Geometry check sheet. Reference: the model listing, model coordinates, mm. Face numbers are marked on the shaded views. A direction names the side the tool comes from. Round coordinates to 2 decimals unless told otherwise and drop trailing zeros. Order: outer loops, then holes, each group sorted by start corner. A loop starts at its lowest first (then second) coordinate and runs counter-clockwise, first axis right, second up. Notation, with made-up numbers: (74, 74.5) - (94, 74.5) arc R23 cw to (94, 102.5) - close; hole circle Ø4 at (4, 40.5). An arc over 180 degrees is marked (long way). One line per question, with ' | ' between items. Start each with the question number.
Q1. Tool access check on the marked faces 1, 2 and 3. Record the directions out of +Z, -Z, +X, -X, +Y, -Y that give a thin tool (end or side, any length) a straight path to the whole face; none if there is none.
Q2. Gauge pin test, flat ends, axial feed: P1, Ø9.5, axis at x = 0, y = 0, coming from the -Z side; P2, Ø0.9, axis at y = 7.5, z = 1.5, coming from the -X side; P3, Ø3, axis at x = -5.17, y = 8.85, coming from the +Z side; P4, Ø5, axis at x = 0, y = 0, coming from the +Z side. Record the tip position at first contact, or that the pin passes through.
Q3. Material ranges on line 1 along Y through (x, z) = (0, 2.8); line 2 along Y through (x, z) = (0, 0.3); line 3 along X through (y, z) = (-10.5, 2.75), recorded low to high.
Q4. Sectioned sample at B-B, the plane y = -17.5. Enter the section's corners in (x, z), then the cut area to 3 significant figures.
Q5. Sectioned sample at D-D, the plane y = 0. Give the number of separate pieces and of enclosed holes in the cut face, then the cut area to 3 significant figures.
Q6. Sectioned sample at A-A, the plane x = 0. Enter the section's corners in (y, z).
Q7. Sectioned sample at C-C, the plane z = 1.85. Enter the section's corners in (x, y) (3 decimals).
Q8. Mould release check, pull along Y, two halves, no side actions. Record for the marked faces 4, 5, 6 and 7: +Y half, -Y half, draft (parallel to the pull), parting line (faces both ways), or undercut.
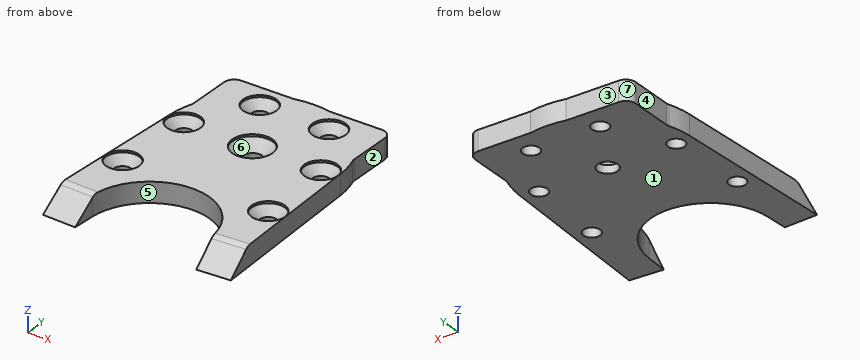
```python
from build123d import *

# Parameters (mm, degrees)
SKETCH1_R                                      = 1.25
SKETCH1_R_2                                    = 1.5
BOSS_EXTRUDE1_DEPTH                            = 3
CSK_FOR_M2_5_FLAT_HEAD_MACHINE_SCREW2_AT_COUNT = 2
CSK_FOR_M2_5_FLAT_HEAD_MACHINE_SCREW2_AT_PITCH = 10.201972061
CSK_FOR_M2_5_FLAT_HEAD_MACHINE_SCREW_2_COUNT   = 2
CSK_FOR_M2_5_FLAT_HEAD_MACHINE_SCREW_2_PITCH   = 17.781163237
CSK_FOR_M2_5_FLAT_HEAD_MACHINE_SCREW_3_COUNT   = 2
CSK_FOR_M2_5_FLAT_HEAD_MACHINE_SCREW_3_PITCH   = 20.5
CSK_FOR_M2_5_FLAT_HEAD_MACHINE_SCREW_4_COUNT   = 2
CSK_FOR_M2_5_FLAT_HEAD_MACHINE_SCREW_4_PITCH   = 12
CSK_FOR_M2_5_FLAT_HEAD_MACHINE_SCREW_5_COUNT   = 2
CSK_FOR_M2_5_FLAT_HEAD_MACHINE_SCREW_5_PITCH   = 24.295707673
CUT_EXTRUDE4_REACH                             = 38.909
CUT_EXTRUDE5_REACH                             = 38.909
FILLET2_R                                      = 1.5


with BuildPart() as part:
    # Sketch1 → Boss-Extrude1 (new body)
    with BuildSketch(Plane.XY):
        with BuildLine():
            ThreePointArc((12.078947368, 4.081853803), (12.019868427, 4.318739766), (12, 4.562071898))
            Line((12, 4.562071898), (12, 10.970231229))
            ThreePointArc((12, 10.970231229), (11.560660172, 12.030891401), (10.5, 12.470231229))
            Line((10.5, 12.470231229), (2.656281818, 12.470231229))
            ThreePointArc((2.656281818, 12.470231229), (0, 12.75), (-2.656281818, 12.470231229))
            Line((-2.656281818, 12.470231229), (-10.5, 12.470231229))
            ThreePointArc((-10.5, 12.470231229), (-11.560660172, 12.030891401), (-12, 10.970231229))
            Line((-12, 10.970231229), (-12, 4.562071898))
            ThreePointArc((-12, 4.562071898), (-12.019868427, 4.318739766), (-12.078947368, 4.081853803))
            ThreePointArc((-12.078947368, 4.081853803), (-12.522664749, 2.396949642), (-12.732526568, 0.667283442))
            Line((-12.732526568, 0.667283442), (-14.040925474, -24.298454927))
            Line((-14.040925474, -24.298454927), (-9.0477778, -24.560134708))
            Line((-9.0477778, -24.560134708), (-8.869966, -21.167283442))
            ThreePointArc((-8.869966, -21.167283442), (0, -12.75), (8.869966, -21.167283442))
            Line((8.869966, -21.167283442), (9.0477778, -24.560134708))
            Line((9.0477778, -24.560134708), (14.040925474, -24.298454927))
            Line((14.040925474, -24.298454927), (12.732526568, 0.667283442))
            ThreePointArc((12.732526568, 0.667283442), (12.522664749, 2.396949642), (12.078947368, 4.081853803))
        make_face()
        with Locations((5.172915418, 8.848923442)):
            Circle(SKETCH1_R, mode=Mode.SUBTRACT)
        with Locations((10.25, 0)):
            Circle(SKETCH1_R, mode=Mode.SUBTRACT)
        with Locations((10.884912472, -11.983191818)):
            Circle(SKETCH1_R, mode=Mode.SUBTRACT)
        Circle(SKETCH1_R_2, mode=Mode.SUBTRACT)
        with Locations((-10.25, 0)):
            Circle(SKETCH1_R, mode=Mode.SUBTRACT)
        with Locations((-5.172915418, 8.848923442)):
            Circle(SKETCH1_R, mode=Mode.SUBTRACT)
        with Locations((-10.884912472, -11.983191818)):
            Circle(SKETCH1_R, mode=Mode.SUBTRACT)
    extrude(amount=BOSS_EXTRUDE1_DEPTH)

    # Sketch3 → CSK for M3 Flat Head Machine Screw1 (revolve, cut)
    with BuildSketch(Plane(origin=(0, 0, 3), x_dir=(0, -1, 0), z_dir=(1, 0, 0))):
        Polygon((0, 0), (0, 5.901290929), (1.5, 5), (1.5, 1.8), (3, 0.3), (3, 0), align=None)
    revolve(axis=Axis((0, 0, 9.35), (0, 0, -1)), mode=Mode.SUBTRACT)

    # Sketch6 → CSK for M2.5 Flat Head Machine Screw2 (revolve, cut)
    with BuildSketch(Plane(origin=(-10.25, 0, 3), x_dir=(0, -1, 0), z_dir=(1, 0, 0))):
        Polygon((0, 0), (0, 5.751075774), (1.25, 5), (1.25, 1.525), (2.475, 0.3), (2.475, 0), align=None)
    csk_for_m2_5_flat_head_machine_screw2 = revolve(axis=Axis((-10.25, 0, 9.35), (0, 0, -1)), mode=Mode.SUBTRACT)

    # CSK for M2.5 Flat Head Machine Screw2 at: CSK for M2.5 Flat Head Machine Screw2 ×2
    with Locations(*[Vector(0.4976571736965763, 0.8673738164530538, 0) * (i * CSK_FOR_M2_5_FLAT_HEAD_MACHINE_SCREW2_AT_PITCH) for i in range(1, CSK_FOR_M2_5_FLAT_HEAD_MACHINE_SCREW2_AT_COUNT)]):
        add(csk_for_m2_5_flat_head_machine_screw2, mode=Mode.SUBTRACT)

    # CSK for M2.5 Flat Head Machine Screw 2: CSK for M2.5 Flat Head Machine Screw2 ×2
    with Locations(*[Vector(0.8673738164530539, 0.497657173696576, 0) * (i * CSK_FOR_M2_5_FLAT_HEAD_MACHINE_SCREW_2_PITCH) for i in range(1, CSK_FOR_M2_5_FLAT_HEAD_MACHINE_SCREW_2_COUNT)]):
        add(csk_for_m2_5_flat_head_machine_screw2, mode=Mode.SUBTRACT)

    # CSK for M2.5 Flat Head Machine Screw 3: CSK for M2.5 Flat Head Machine Screw2 ×2
    with Locations(*[(i * CSK_FOR_M2_5_FLAT_HEAD_MACHINE_SCREW_3_PITCH, 0, 0) for i in range(1, CSK_FOR_M2_5_FLAT_HEAD_MACHINE_SCREW_3_COUNT)]):
        add(csk_for_m2_5_flat_head_machine_screw2, mode=Mode.SUBTRACT)

    # CSK for M2.5 Flat Head Machine Screw 4: CSK for M2.5 Flat Head Machine Screw2 ×2
    with Locations(*[Vector(-0.05290937262723391, -0.9985993181893289, 0) * (i * CSK_FOR_M2_5_FLAT_HEAD_MACHINE_SCREW_4_PITCH) for i in range(1, CSK_FOR_M2_5_FLAT_HEAD_MACHINE_SCREW_4_COUNT)]):
        add(csk_for_m2_5_flat_head_machine_screw2, mode=Mode.SUBTRACT)

    # CSK for M2.5 Flat Head Machine Screw 5: CSK for M2.5 Flat Head Machine Screw2 ×2
    with Locations(*[Vector(0.8699031432206916, -0.4932225881027359, 0) * (i * CSK_FOR_M2_5_FLAT_HEAD_MACHINE_SCREW_5_PITCH) for i in range(1, CSK_FOR_M2_5_FLAT_HEAD_MACHINE_SCREW_5_COUNT)]):
        add(csk_for_m2_5_flat_head_machine_screw2, mode=Mode.SUBTRACT)

    # Sketch10 → Cut-Extrude4 (cut, up to next)
    with BuildSketch(Plane(origin=(12.732526568, 0.667283442, 0), x_dir=(0, 0, -1), z_dir=(0.9986295347545739, 0.052335956242944286, 0)), mode=Mode.PRIVATE) as cut_extrude4_sk1:
        Polygon((-3, -25), (0, -25), (-3, -21.113156261), align=None)
    cut_extrude4_tool1 = extrude(cut_extrude4_sk1.sketch, amount=-CUT_EXTRUDE4_REACH, mode=Mode.PRIVATE) & part.part
    add(cut_extrude4_tool1.solids().sort_by_distance((13.973118, -23.004616, 2))[0], mode=Mode.SUBTRACT)

    # Sketch11 → Cut-Extrude5 (cut, up to next)
    with BuildSketch(Plane(origin=(-12.732526568, 0.667283442, 0), x_dir=(0, 0, 1), z_dir=(-0.9986295347545739, 0.052335956242944716, 0)), mode=Mode.PRIVATE) as cut_extrude5_sk1:
        Polygon((3, -21.113156261), (0, -25), (3, -25), align=None)
    cut_extrude5_tool1 = extrude(cut_extrude5_sk1.sketch, amount=-CUT_EXTRUDE5_REACH, mode=Mode.PRIVATE) & part.part
    add(cut_extrude5_tool1.solids().sort_by_distance((-13.973118, -23.004616, 2))[0], mode=Mode.SUBTRACT)

    # Fillet2
    fillet2_edges = [part.edges().sort_by_distance(p)[0] for p in [
        (11.334194425, -20.548130857, 3),
        (-11.334194425, -20.548130857, 3),
    ]]
    fillet(fillet2_edges, radius=FILLET2_R)


solid = part.part
```
Determined:
1) face 1: -Z, +X, -X, +Y, -Y | face 2: +Z, -Z, +X, +Y | face 3: +Z, -Z, -X, +Y
2) P1: stops at z = 0 | P2: stops at x = -12 | P3: stops at z = 1.73 | P4: stops at z = 2.2
3) line 1: y = -12.75 to -3, 3 to 12.75 | line 2: y = -12.75 to -1.5, 1.5 to 12.75 | line 3: x = -13.32 to -12.87, -8.9 to 8.9, 12.87 to 13.32
4) outline: (-13.68, 0) - (-7.86, 0) - (-7.86, 3) - (-13.68, 3) - close; (7.86, 0) - (13.68, 0) - (13.68, 3) - (7.86, 3) - close | area: 34.9 mm2
5) separate pieces: 4 | enclosed holes: 0 | area: 45.0 mm2
6) outline: (-12.75, 0) - (-1.5, 0) - (-1.5, 1.2) - (-3, 2.7) - (-3, 3) - (-12.75, 3) - close; (1.5, 0) - (12.75, 0) - (12.75, 3) - (3, 3) - (3, 2.7) - (1.5, 1.2) - close
7) outline: (-13.915, -21.905) - (-8.922, -22.167) - (-8.87, -21.167) arc R8.882 cw to (8.87, -21.167) - (8.922, -22.167) - (13.915, -21.905) - (12.733, 0.667) arc R12.75 ccw to (12.079, 4.082) arc R1.5 cw to (12, 4.562) - (12, 10.97) arc R1.5 ccw to (10.5, 12.47) - (2.656, 12.47) arc R12.75 ccw to (-2.656, 12.47) - (-10.5, 12.47) arc R1.5 ccw to (-12, 10.97) - (-12, 4.562) arc R1.5 cw to (-12.079, 4.082) arc R12.75 ccw to (-12.733, 0.667) - close; hole circle Ø3.25 at (-10.885, -11.983); hole circle Ø3.25 at (-10.25, 0); hole circle Ø3.25 at (-5.173, 8.849); hole circle Ø4.3 at (0, 0); hole circle Ø3.25 at (5.173, 8.849); hole circle Ø3.25 at (10.25, 0); hole circle Ø3.25 at (10.885, -11.983)
8) face 4: draft | face 5: -Y half | face 6: undercut | face 7: +Y half
